from build123d import *

# Parameters (mm, degrees)
PAD_DEPTH       = 20
SKETCH001_W     = 19.994943
SKETCH001_H     = 14
POCKET_DEPTH    = 20
SKETCH002_R     = 2.5
POCKET001_DEPTH = 5
SKETCH003_R     = 2.5
POCKET002_DEPTH = 5


with BuildPart() as part:
    # Sketch → Pad (new body)
    with BuildSketch(Plane.XZ):
        Polygon((-51.993317, 0), (-51.993317, 24.000334), (-47.994495, 24.000334), (-27.999552, 3.999817), (-27.999552, 0), align=None)
    extrude(amount=PAD_DEPTH)

    # Sketch001 → Pocket (cut)
    with BuildSketch(Plane(origin=(0, 0, 24.000334), x_dir=(-1, 0, 0), z_dir=(0, 0, 1))):
        with Locations((37.9970235, 10)):
            Rectangle(SKETCH001_W, SKETCH001_H)
    extrude(amount=-POCKET_DEPTH, mode=Mode.SUBTRACT)

    # Sketch002 → Pocket001 (cut)
    with BuildSketch(Plane(origin=(-47.994495, 0, 0), x_dir=(0, 0, 1), z_dir=(1, 0, 0))):
        with Locations((13.999817, 10)):
            Circle(SKETCH002_R)
    extrude(amount=-POCKET001_DEPTH, mode=Mode.SUBTRACT)

    # Sketch003 → Pocket002 (cut)
    with BuildSketch(Plane(origin=(0, 0, 4.000334), x_dir=(-1, 0, 0), z_dir=(0, 0, 1))):
        with Locations((37.994495, 10)):
            Circle(SKETCH003_R)
    extrude(amount=-POCKET002_DEPTH, mode=Mode.SUBTRACT)


solid = part.part
The listing builds one solid part. Answer for the finished solid, in the listing's coordinates (mm). A direction names the side the tool comes from. Round coordinates to 2 decimals unless told otherwise and drop trailing zeros. Write each loop counter-clockwise with the first axis right and the second up, starting at its lowest first coordinate (ties: lowest second). Pieces come first, ordered by that corner, then holes. Notation, with made-up numbers: (-6.5, 43.25) - (45.5, 43.25) arc R18 cw to (45.5, 69.25) - close; hole circle Ø5 at (-18, -36.75). An arc over 180 degrees is marked (long way). Use one line per item in the form item = value. Start each with the question number.
Item 1: A tool of negligible diameter and unlimited length cuts with its end or side. For faces 5 (the flat face through (-38.784, -17.361, 14.788)), 6 (the flat face through (-40, -12, 4)), from which of +Z, -Z, +X, -X, +Y, -Y can it reach the whole face along a straight path? Write none if from no direction.
Item 2: A cutting plane is placed at D-D (x = -30.5). Write down the section's boundary in (y, z), plus the area to 3 significant figures.
Item 3: Determine the mould class of faces 1 (the flat face through (-28, -10, 2)), 2 (the cylindrical face through (-36.01, -8.48, 2.03)), 3 (the flat face through (-51.993, -8, 12)), 4 (the flat face through (-42, -20, 10)) for opening direction X: +X half, -X half, draft (parallel to the pull), parting line (faces both ways), or undercut.
Item 4: A cutting plane is placed at B-B (x = -39). Write down the section's boundary in (y, z).
Item 5: Find the intervals of material crossed by line 1 (Y direction, x = -42.5, z = 17.5); line 2 (Z direction, x = -48.8, y = -10); line 3 (X direction, y = -10, z = 2.15), in increasing order. Write a range as [from, to].
Item 6: Flat-ended cylindrical pins translate along their axes: pin 1 Ø6 at (x, z) = (-36, 15.5) entering from +Y; pin 2 Ø3 at (x, y) = (-42, -2) entering from +Z. Find the tip coordinate at first contact, or state that the pin passes through.
Item 7: A cutting plane is placed at A-A (y = -10). Give the number of separate pieces and of enclosed holes in the cut face, plus the area to 3 significant figures.
The answers:
q1.face_5 = +Z, +X, +Y, -Y
q1.face_6 = +Z, +X
q2.outline = (-20, 0) - (0, 0) - (0, 6.5) - (-3, 6.5) - (-3, 4) - (-17, 4) - (-17, 6.5) - (-20, 6.5) - close
q2.area = 95.0 mm^2
q3.face_1 = +X half
q3.face_2 = undercut
q3.face_3 = -X half
q3.face_4 = draft
q4.outline = (-20, 0) - (-12.29, 0) - (-12.29, 4) - (-17, 4) - (-17, 15) - (-20, 15) - close; (-7.71, 0) - (0, 0) - (0, 15) - (-3, 15) - (-3, 4) - (-7.71, 4) - close
q5.line_1 = [-20, -17], [-3, 0]
q5.line_2 = [0, 11.5], [16.5, 24]
q5.line_3 = [-51.99, -40.49], [-35.49, -28]
q6.pin_1 = 0
q6.pin_2 = 19.5
q7.separate_pieces = 3
q7.enclosed_holes = 0
q7.area = 136 mm^2
